Autodesk Fusion 360 part; units mm, degrees
sketch "Sketch1" plane through (0, 0, 0) normal (0, 0, 1) x (1, 0, 0)
  circle A0 centre (0.4513, 0) radius 4
  dimension "d1" = 8
extrude "Extrude1" add sketch "Sketch1" along normal blind 4
sketch "Sketch2" plane through (0, 0, 4) normal (0, 0, 1) x (-1, 0, 0)
  circle A0 centre (-0.4513, 0) radius 4
  circle A1 centre (-0.4513, 0) radius 3.5
  circle A2 centre (-0.4513, 0) radius 0.625
  dimension "d4" = 7
  dimension "d5" = 1.25
extrude "Extrude2" cut 1 faces at (2.3843, -0.8657, 4) along direction (0, 0, -1) blind 1
loft "Loft1" add profiles "Sketch2" section 1 face at (2.3843, -0.8657, 3) section 2 contours A1
extrude "Extrude3" add sketch "Sketch2" along normal blind 2 contours A2
Part model, mm, in its own coordinate system. A direction names the side the tool comes from. Round coordinates to 2 decimals unless told otherwise and drop trailing zeros. Write each loop counter-clockwise with the first axis right and the second up, starting at its lowest first coordinate (ties: lowest second). Pieces come first, ordered by that corner, then holes. Notation, with made-up numbers: (-13.5, -31) -> (18.5, -31) arc R27 ccw to (18.5, 3) -> close; hole circle Ø5 at (-0.5, 29). An arc over 180 degrees is marked (long way). Return JSON: item names as keys, results as strings. Group by question number.
Q1. Saw through at A-A on z = 5.3. Write the cut outline in (x, y) (3 decimals).
Q2. Saw through at B-B on z = 0.7. Write the cut outline in (x, y), plus the area to 3 significant figures.
Q3. Which spindle directions (+Z, -Z, +X, -X, +Y, -Y) get a long thin tool onto all of the face, cutting with end or side? Do faces 1 (the cylindrical face through (-0.126, -0.239, 4.986)), 2 (the flat face through (0, 0, 6)). Say none if no direction does.
Q4. Pin check, flat tips, straight feed: pin 1 (1.5 mm diameter, centred on y = 1.5, z = 2, fed in from -X); pin 2 (2 mm diameter, centred on y = -2.5, z = 3.5, fed in from -X); pin 3 (3.5 mm diameter, centred on x = 1, y = 1, fed in from +Z); pin 4 (1.5 mm diameter, centred on y = -2, z = 1.5, fed in from +X). Stop position of each tip, or through.
Q5. Probe L1, parallel to Z at x = -0.75, y = 1.5; L2, parallel to Y at x = 0.5, z = 5.3; L3, parallel to Y at x = 2.25, z = 3.7. List the from-to ranges inside material, lowest first. Write a range as [from, to].
Answer:
{
 "1": {"outline": "circle Ø1.25 at (0.451, 0)"},
 "2": {"outline": "circle Ø8 at (0.45, 0)", "area": "50.3 mm2"},
 "3": {"face 1": "+Z", "face 2": "+Z, +X, -X, +Y, -Y"},
 "4": {"pin 1": "x = -3.48", "pin 2": "x = -3.2", "pin 3": "z = 6", "pin 4": "x = 4.25"},
 "5": {"L1": "[0, 4]", "L2": "[-0.62, 0.62]", "L3": "[-3.18, 3.18]"}
}
